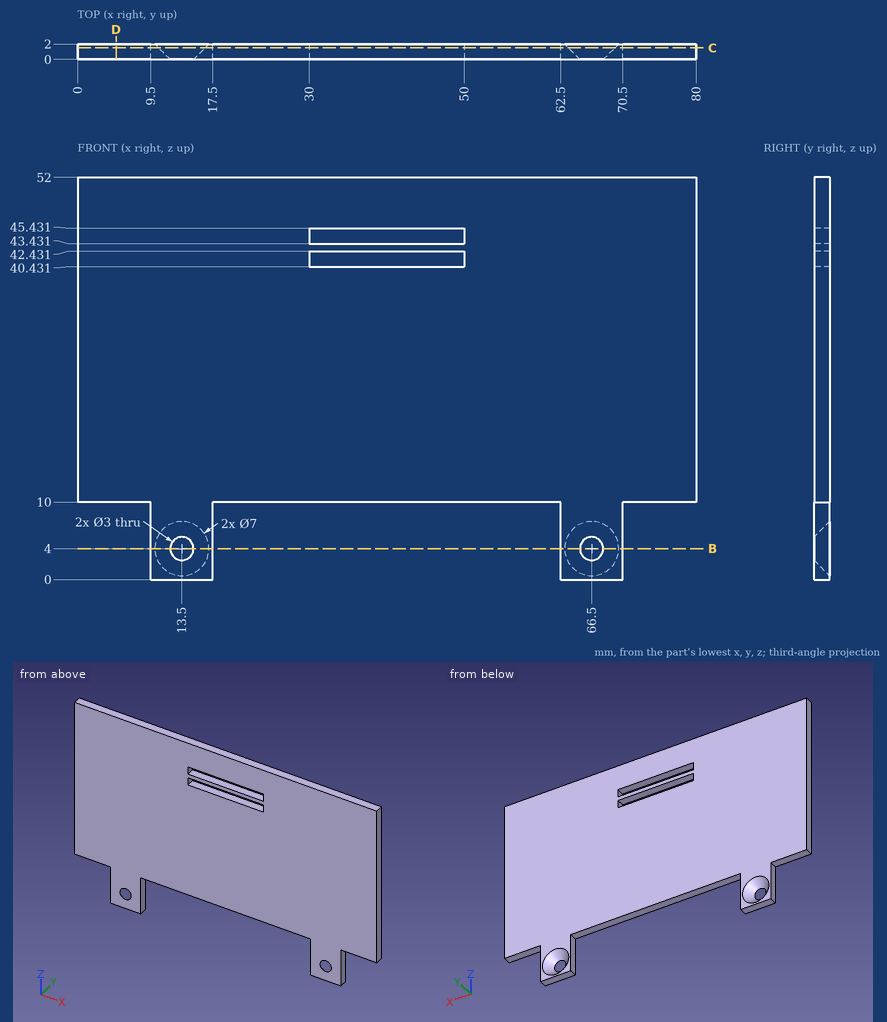
Here's the drawing with two shaded views (mm, measured from the low corner). I have some questions. Coordinates: 2 decimals unless noted, no trailing zeros. Loops run counter-clockwise (first coordinate to the right, second up) from the corner with the lowest first, then second, coordinate; pieces in that order, holes last. Notation, with made-up numbers: (-16.75, -23) -> (11.25, -23) arc R27 ccw to (11.25, 4) -> close; hole circle Ø4 at (-29.75, 11.25). An arc over 180 degrees is marked (long way). Put each result on its own line as item: value. Start each with the question number.
Q1. If I drill on line 1 (Z direction, x = 36, y = 0.6); line 2 (X direction, y = 0.4, z = 42); line 3 (X direction, y = 1.25, z = 9.5), over which ranges is the centre line in solid material (lowest first)? Write a range as [from, to].
Q2. I want a section at B-B (z = 4). Count the separate pieces of the cut face and the enclosed holes in it, plus the area to 3 significant figures.
Q3. I want a section at D-D (x = 5). Write out the boundary of the cut face in (y, z).
Q4. I want a section at C-C (y = 1.5). Write out the boundary of the cut face in (x, z).
Q5. I'm going to push flat-ended pins straight in: P1, Ø1, axis at y = 1, z = 45, coming from the -X side; P2, Ø0.6, axis at y = 1.5, z = 5, coming from the +X side; P3, Ø1.8, axis at x = 13.5, z = 4, coming from the +Y side; P4, Ø5, axis at x = 66.5, z = 4, coming from the +Y side. Where does each tip first touch, or does it pass through?
Taken from the geometry:
1. line 1: z = [10, 40.43], [42.43, 43.43], [45.43, 52]
1. line 2: x = [0, 30], [50, 80]
1. line 3: x = [9.5, 17.5], [62.5, 70.5]
2. separate pieces: 4
2. enclosed holes: 0
2. area: 12.0 mm2
3. outline: (0, 10) -> (2, 10) -> (2, 52) -> (0, 52) -> close
4. outline: (0, 10) -> (9.5, 10) -> (9.5, 0) -> (17.5, 0) -> (17.5, 10) -> (62.5, 10) -> (62.5, 0) -> (70.5, 0) -> (70.5, 10) -> (80, 10) -> (80, 52) -> (0, 52) -> close; hole circle Ø6 at (13.5, 4); hole (30, 40.43) -> (50, 40.43) -> (50, 42.43) -> (30, 42.43) -> close; hole (30, 43.43) -> (50, 43.43) -> (50, 45.43) -> (30, 45.43) -> close; hole circle Ø6 at (66.5, 4)
5. P1: stops at x = 0
5. P2: stops at x = 70.5
5. P3: passes through
5. P4: stops at y = 1
